The listing builds one solid part. Answer for the finished solid, in the listing's coordinates (mm). Face numbers are marked on the shaded views. A direction names the side the tool comes from. Round coordinates to 2 decimals unless told otherwise and drop trailing zeros. Order: outer loops, then holes, each group sorted by start corner. A loop starts at its lowest first (then second) coordinate and runs counter-clockwise, first axis right, second up. Notation, with made-up numbers: (-18.75, 0) -> (4.25, 0) arc R19 cw to (4.25, 19) -> close; hole circle Ø1 at (-2.5, 70). An arc over 180 degrees is marked (long way). Return JSON: item names as keys, results as strings. Group by question number.
(1) Determine the mould class of the marked faces 1, 2, 3 and 4 for opening direction X: +X half, -X half, draft (parallel to the pull), parting line (faces both ways), or undercut.
(2) Consider line 1 (X direction, y = 51.5, z = 24); line 2 (Y direction, x = 19, z = 21.75); line 3 (Y direction, x = -55, z = 27.25). Determine where each line is inside the solid, lowest interval first. Write a range as [from, to].
(3) Which of the six approach directions +Z, -Z, +X, -X, +Y, -Y give full straight-line access (tool end or side, diameter ignored) to the marked faces 5, 6 and 7?
(4) The part is cut by section D-D (x = 125.5). Determine the outline of the cut face in (y, z).
(5) Each of these flat-tipped pins is pushed along its axis until it touches: pin 1 (15 mm diameter, centred on x = 8.5, z = 21.5, fed in from +Y); pin 2 (1.5 mm diameter, centred on x = 253.5, z = 13, fed in from -Y). Where does it stop, or does it pass through?
(6) The part is cut by section C-C (x = 229). Determine the outline of the cut face in (y, z), plus the area to 3 significant figures.
(7) The part is cut by section A-A (y = 177). Determine the outline of the cut face in (x, z).
from build123d import *

# Parameters (mm, degrees)
EXTRUDE_1_DEPTH     = 30
FILLET_1_R          = 15
FILLET_2_R          = 30
CUT_EXTRUDE_1_DEPTH = 30
CUT_EXTRUDE_2_DEPTH = 40


with BuildPart() as part:
    # 草图1 → 凸台-拉伸1 (new body)
    with BuildSketch(Plane.XY):
        with BuildLine():
            Line((-323, 208), (-323, 33))
            Line((-323, 33), (-183, 33))
            Line((-183, 33), (-150, 0))
            Line((-150, 0), (150, 0))
            Line((150, 0), (183, 33))
            Line((183, 33), (323, 33))
            Line((323, 33), (323, 208))
            Line((323, 208), (203, 208))
            Line((203, 208), (189.154352992, 150.927256427))
            ThreePointArc((189.154352992, 150.927256427), (178.544779492, 134.418414947), (160, 128))
            Line((160, 128), (-160, 128))
            ThreePointArc((-160, 128), (-178.544779492, 134.418414947), (-189.154352992, 150.927256427))
            Line((-189.154352992, 150.927256427), (-203, 208))
            Line((-203, 208), (-323, 208))
        make_face()
    extrude(amount=EXTRUDE_1_DEPTH)

    # 圆角1
    fillet_1_edges = [part.edges().sort_by_distance(p)[0] for p in [
        (-203, 208, 15),
        (203, 208, 15),
        (323, 208, 15),
        (323, 33, 15),
        (-323, 33, 15),
        (-323, 208, 15),
    ]]
    fillet(fillet_1_edges, radius=FILLET_1_R)

    # 圆角2
    fillet_2_edges = [part.edges().sort_by_distance(p)[0] for p in [
        (183, 33, 15),
        (150, 0, 15),
        (-150, 0, 15),
        (-183, 33, 15),
    ]]
    fillet(fillet_2_edges, radius=FILLET_2_R)

    # 草图2 → 切除-拉伸1 (cut)
    with BuildSketch(Plane.XY.offset(30)):
        with BuildLine():
            Line((-24, 88), (24, 88))
            ThreePointArc((24, 88), (31.071067812, 85.071067812), (34, 78))
            Line((34, 78), (34, 30))
            ThreePointArc((34, 30), (31.071067812, 22.928932188), (24, 20))
            Line((24, 20), (-24, 20))
            ThreePointArc((-24, 20), (-31.071067812, 22.928932188), (-34, 30))
            Line((-34, 30), (-34, 78))
            ThreePointArc((-34, 78), (-31.071067812, 85.071067812), (-24, 88))
        make_face()
    extrude(amount=-CUT_EXTRUDE_1_DEPTH, mode=Mode.SUBTRACT)

    # 草图3 → 切除-拉伸2 (cut, symmetric)
    with BuildSketch(Plane(origin=(0, 0, 0), x_dir=(0, 0, -1), z_dir=(1, 0, 0))):
        Polygon((0, 130), (-12, 130), (0, 110), align=None)
    extrude(amount=CUT_EXTRUDE_2_DEPTH, both=True, mode=Mode.SUBTRACT)


solid = part.part
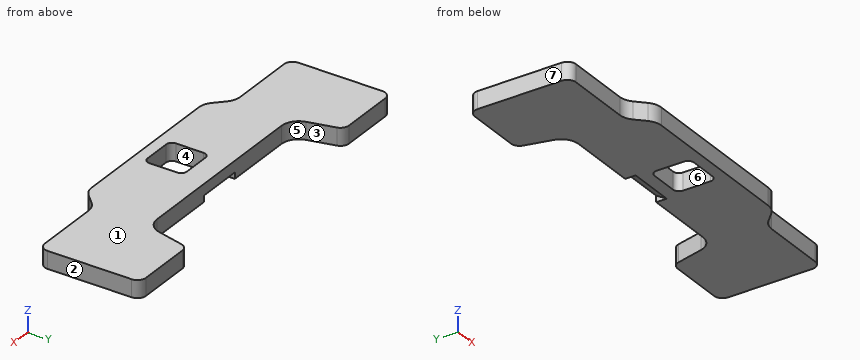
Answer below:
{
 "1": {"face 1": "draft", "face 2": "+X half", "face 3": "undercut", "face 4": "undercut"},
 "2": {"line 1": "x = [-323, -34], [34, 323]", "line 2": "y = [0, 20], [88, 128]", "line 3": "y = [0, 128]"},
 "3": {"face 5": "+Z, -Z, +Y", "face 6": "+Z, -Z", "face 7": "+Z, -Z, -X, +Y, -Y"},
 "4": {"outline": "(0, 0) -> (128, 0) -> (128, 30) -> (0, 30) -> close"},
 "5": {"pin 1": "stops at y = 128", "pin 2": "stops at y = 33"},
 "6": {"outline": "(33, 0) -> (208, 0) -> (208, 30) -> (33, 30) -> close", "area": "5,250 mm²"},
 "7": {"outline": "(-323, 0) -> (-195.48, 0) -> (-195.48, 30) -> (-323, 30) -> close; (195.48, 0) -> (323, 0) -> (323, 30) -> (195.48, 30) -> close"}
}
